from build123d import *

# Parameters (mm, degrees)
F0_W      = 152.0007625222
F0_H      = 150.7072374225
F1_DEPTH  = 76.2
F3_DEPTH  = 76.2
F4_DEPTH  = 1270
F6_DEPTH  = 25.4
F7_W      = 24.8957742006
F7_H      = 18.5917448044
F8_DEPTH  = 1270
F10_DEPTH = 152.0017625222


with BuildPart() as f1:
    # F0 (on Top) → F1 (new body)
    with BuildSketch(Plane.XY):
        with Locations((0.2458952367, 0.141967088)):
            Rectangle(F0_W, F0_H)
    extrude(amount=F1_DEPTH)

    # F2 (on face) → F3 (cut)
    with BuildSketch(Plane.XZ.offset(75.2116516232)):
        Polygon((76.2462764978, 76.2), (0, 76.2), (76.2462764978, 0), align=None)
    extrude(amount=-F3_DEPTH, mode=Mode.SUBTRACT)

    # F4 (cut): a face of the model
    f4_faces = [f1.faces().sort_by_distance(p)[0] for p in [
        (50.8308509986, 0.9883483768, 50.8),
    ]]
    extrude(f4_faces, amount=-F4_DEPTH, mode=Mode.SUBTRACT)

    # F5 (on face) → F6 (join)
    with BuildSketch(Plane.XZ.offset(75.2116516232)):
        Polygon((0, 76.2), (-10.1499548182, 76.2), (-10.1499548182, 0), (14.0455085784, 0), (14.0455085784, 62.1630161257), align=None)
    extrude(amount=F6_DEPTH)

    # F7 (on face) → F8 (cut)
    with BuildSketch(Plane(origin=(-75.7544860244, 0, 0), x_dir=(0, -1, 0), z_dir=(-1, 0, 0))):
        with Locations((0, 66.9041275978)):
            Rectangle(F7_W, F7_H)
    extrude(amount=-F8_DEPTH, mode=Mode.SUBTRACT)

    # F9 (on face) → F10 (cut, through all)
    with BuildSketch(Plane(origin=(-75.7544860244, 0, 0), x_dir=(0, -1, 0), z_dir=(-1, 0, 0))):
        with BuildLine():
            Line((-57.8758810088, 47.2911335528), (-32.2743262723, 47.2911335528))
            ThreePointArc((-32.2743262723, 47.2911335528), (-45.0751036406, 60.091910921), (-57.8758810088, 47.2911335528))
        make_face()
        with BuildLine():
            ThreePointArc((-57.8758810088, 47.2911335528), (-45.0751036406, 34.4903561846), (-32.2743262723, 47.2911335528))
            Line((-32.2743262723, 47.2911335528), (-57.8758810088, 47.2911335528))
        make_face()
        with BuildLine():
            Line((-58.0906374395, 14.1140213236), (-32.4261682093, 14.1140213236))
            ThreePointArc((-32.4261682093, 14.1140213236), (-45.2584028244, 26.9462559387), (-58.0906374395, 14.1140213236))
        make_face()
        with BuildLine():
            ThreePointArc((-58.0906374395, 14.1140213236), (-45.2584028244, 1.2817867085), (-32.4261682093, 14.1140213236))
            Line((-32.4261682093, 14.1140213236), (-58.0906374395, 14.1140213236))
        make_face()
        with BuildLine():
            ThreePointArc((32.553633581, 14.1140213236), (45.4745851457, 1.1930697589), (58.3955367104, 14.1140213236))
            Line((58.3955367104, 14.1140213236), (32.553633581, 14.1140213236))
        make_face()
        with BuildLine():
            Line((32.553633581, 14.1140213236), (58.3955367104, 14.1140213236))
            ThreePointArc((58.3955367104, 14.1140213236), (45.4745851457, 27.0349728883), (32.553633581, 14.1140213236))
        make_face()
        with BuildLine():
            ThreePointArc((32.6371107909, 47.2911335528), (45.4745851457, 34.453659198), (58.3120595005, 47.2911335528))
            Line((58.3120595005, 47.2911335528), (32.6371107909, 47.2911335528))
        make_face()
        with BuildLine():
            Line((32.6371107909, 47.2911335528), (58.3120595005, 47.2911335528))
            ThreePointArc((58.3120595005, 47.2911335528), (45.4745851457, 60.1286079076), (32.6371107909, 47.2911335528))
        make_face()
    extrude(amount=-F10_DEPTH, mode=Mode.SUBTRACT)


solid = f1.part
CAD build for the part. Positions are in the model's coordinates, mm. A direction names the side the tool comes from. Round coordinates to 2 decimals unless told otherwise and drop trailing zeros. Write each loop counter-clockwise with the first axis right and the second up, starting at its lowest first coordinate (ties: lowest second). Pieces come first, ordered by that corner, then holes. Notation, with made-up numbers: M 49,81 L 54,81 A15 cw 54,97 Z; hole C 74.25,62 d1. An arc over 180 degrees is marked long. Use a Markdown table: item, result. Add a question column.
1. Slice it at A-A on z = 52.5. Give the cut face in (x, y), then the cut area to 3 significant figures.
2. Pull direction Z, two halves, no side cores. Call faces 1 (the face through (38.657, -11.325, 37.567)), 2 (the face through (-1.45, 52.157, 3.294)), 3 (the face through (-75.754, -1, 38)): released by +Z, released by -Z, zero draft, split by the parting line, or undercut.
3. Flat gauge pins, fed straight in: P1, Ø6, axis at x = 19, z = 24, coming from the -Y side; P2, Ø10, axis at x = 56.5, y = -46, coming from the +Z side; P3, Ø12.5, axis at y = -86, z = 41, coming from the -X side. Where does each tip first touch, or does it go through?
4. 3-axis set-ups, long thin cutter, end or side, ignore diameter. For faces 4 (the face through (-1, -11, 0)), 5 (the face through (14.046, -88, 31)), 6 (the face through (-29, -12.448, 67)), 7 (the face through (-10.15, -88, 39)): which of +Z, -Z, +X, -X, +Y, -Y reach the whole face in a straight line?
5. Slice it at B-B on y = 53. Give the cut face in (x, z).
6. Slice it at D-D on z = 69.5. Give the cut face in (x, y), then the cut area to 3 significant figures.
7. Drill centre lines: probe 1 along Y at (x, z) = (-68.5, 66.5); probe 2 along Y at (x, z) = (-36, 46.5); probe 3 along Y at (x, z) = (-42, 23). Where is each one in solid material? Low to high.
8. Slice it at C-C on x = -63. Give the cut face in (y, z).
Reply:
| question | item | result |
|---|---|---|
| 1 | outline | M -75.75,-75.21 L -10.15,-75.21 L -10.15,-100.61 L 14.05,-100.61 L 14.05,-75.21 L 23.71,-75.21 L 23.71,-57.21 L -75.75,-57.21 Z; M -75.75,-33.74 L 23.71,-33.74 L 23.71,33.38 L -75.75,33.38 Z; M -75.75,56.77 L 23.71,56.77 L 23.71,75.5 L -75.75,75.5 Z |
| 1 | area | 10,900 mm^2 |
| 2 | face 1 | released by +Z |
| 2 | face 2 | undercut |
| 2 | face 3 | zero draft |
| 3 | P1 | stops at y = -75.21 |
| 3 | P2 | stops at z = 2.43 |
| 3 | P3 | stops at x = -10.15 |
| 4 | face 4 | -Z, +X, -X, +Y, -Y |
| 4 | face 5 | +Z, -Z, +X, -Y |
| 4 | face 6 | +Z, +X, -X |
| 4 | face 7 | +Z, -Z, -X, -Y |
| 5 | outline | M -75.75,0 L 76.25,0 L 72.36,3.88 L -75.75,3.88 Z; M -75.75,24.35 L 51.88,24.35 L 38.99,37.24 L -75.75,37.24 Z; M -75.75,57.34 L 18.87,57.34 L 0,76.2 L -75.75,76.2 Z |
| 6 | outline | M -75.75,-75.21 L -10.15,-75.21 L -10.15,-100.61 L 6.7,-100.61 L 6.7,-12.45 L -75.75,-12.45 Z; M -75.75,12.45 L 6.7,12.45 L 6.7,75.5 L -75.75,75.5 Z |
| 6 | area | 10,800 mm^2 |
| 7 | probe 1 | y = -75.21 to -12.45, 12.45 to 75.5 |
| 7 | probe 2 | y = -75.21 to -58.29, -32.66 to 32.3, 57.85 to 75.5 |
| 7 | probe 3 | y = -75.21 to -54.85, -36.09 to 36, 54.52 to 75.5 |
| 8 | outline | M -75.21,0 L 75.5,0 L 75.5,76.2 L 12.45,76.2 L 12.45,57.61 L -12.45,57.61 L -12.45,76.2 L -75.21,76.2 Z; hole C -45.47,14.11 d25.84; hole C -45.47,47.29 d25.67; hole C 45.08,47.29 d25.6; hole C 45.26,14.11 d25.66 |
